from build123d import *

# Parameters (mm, degrees)
F0_R     = 11.425
F1_DEPTH = 8


with BuildPart() as f1:
    # F0 (on Front) → F1 (new body)
    with BuildSketch(Plane.XZ):
        with BuildLine():
            ThreePointArc((-40.4296863013, -48.1120131359), (-39.1212964763, -51.0311038498), (-38.6734638929, -54.1985034943))
            ThreePointArc((-38.6734638929, -54.1985034943), (-53.2658635374, -65.1756709109), (-59.7672414846, -48.1120131359))
            Line((-59.7672414846, -48.1120131359), (-65.0984638929, -49.8442323013))
            Line((-65.0984638929, -49.8442323013), (-65.0984638929, -54.1985034943))
            ThreePointArc((-65.0984638929, -54.1985034943), (-50.0984638929, -69.1985034943), (-35.0984638929, -54.1985034943))
            Line((-35.0984638929, -54.1985034943), (-35.0984638929, -49.8442323013))
            Line((-35.0984638929, -49.8442323013), (-40.4296863013, -48.1120131359))
        make_face()
        with BuildLine():
            ThreePointArc((-45.8538077773, -43.5912644821), (-42.7837389166, -45.4220905869), (-40.4296863013, -48.1120131359))
            Line((-40.4296863013, -48.1120131359), (-35.0984638929, -49.8442323013))
            Line((-35.0984638929, -49.8442323013), (-35.0984638929, -44.23865333))
            ThreePointArc((-35.0984638929, -44.23865333), (-36.9292899977, -41.1685844692), (-37.7218056429, -37.6830190937))
            Line((-37.7218056429, -37.6830190937), (-37.9632089773, -38.0152822786))
            ThreePointArc((-37.9632089773, -38.0152822786), (-41.2816851085, -41.3337584099), (-45.4632089773, -43.4643512387))
            Line((-45.4632089773, -43.4643512387), (-45.8538077773, -43.5912644821))
        make_face()
        with BuildLine():
            Line((-65.0984638929, -49.8442323013), (-59.7672414846, -48.1120131359))
            ThreePointArc((-59.7672414846, -48.1120131359), (-57.4131888693, -45.4220905869), (-54.3431200085, -43.5912644821))
            Line((-54.3431200085, -43.5912644821), (-54.7337188086, -43.4643512387))
            ThreePointArc((-54.7337188086, -43.4643512387), (-58.9152426773, -41.3337584099), (-62.2337188086, -38.0152822786))
            Line((-62.2337188086, -38.0152822786), (-62.4751221429, -37.6830190937))
            ThreePointArc((-62.4751221429, -37.6830190937), (-63.2676377882, -41.1685844692), (-65.0984638929, -44.23865333))
            Line((-65.0984638929, -44.23865333), (-65.0984638929, -49.8442323013))
        make_face()
        with BuildLine():
            Line((-35.0984638929, -44.23865333), (-35.0984638929, -49.8442323013))
            Line((-35.0984638929, -49.8442323013), (-30.9573059012, -51.1897760981))
            ThreePointArc((-30.9573059012, -51.1897760981), (-12.0562032411, -41.5591832693), (-21.6867960699, -22.6580806092))
            Line((-21.6867960699, -22.6580806092), (-25.8279540617, -21.3125368125))
            Line((-25.8279540617, -21.3125368125), (-29.1228307116, -25.8475454636))
            ThreePointArc((-29.1228307116, -25.8475454636), (-19.3030867945, -27.9092310939), (-14.8970509856, -36.9239283536))
            ThreePointArc((-14.8970509856, -36.9239283536), (-22.4323140065, -47.6663941429), (-35.0984638929, -44.23865333))
        make_face()
        with BuildLine():
            Line((-69.2396218847, -51.1897760981), (-65.0984638929, -49.8442323013))
            Line((-65.0984638929, -49.8442323013), (-65.0984638929, -44.23865333))
            ThreePointArc((-65.0984638929, -44.23865333), (-84.740697499, -40.4544475144), (-71.0740970743, -25.8475454636))
            Line((-71.0740970743, -25.8475454636), (-74.3689737242, -21.3125368125))
            Line((-74.3689737242, -21.3125368125), (-78.5101317159, -22.6580806092))
            ThreePointArc((-78.5101317159, -22.6580806092), (-88.1407245447, -41.5591832693), (-69.2396218847, -51.1897760981))
        make_face()
        with BuildLine():
            Line((-74.3689737242, -21.3125368125), (-71.0740970743, -25.8475454636))
            ThreePointArc((-71.0740970743, -25.8475454636), (-67.7883864419, -27.255150762), (-65.0984638929, -29.6092033773))
            Line((-65.0984638929, -29.6092033773), (-65.0984638929, -29.1985034943))
            ThreePointArc((-65.0984638929, -29.1985034943), (-64.3643116374, -24.5632485786), (-62.2337188086, -20.3817247099))
            Line((-62.2337188086, -20.3817247099), (-61.9923154742, -20.0494615249))
            ThreePointArc((-61.9923154742, -20.0494615249), (-65.5521859403, -20.3728332923), (-69.0377513159, -19.580317647))
            Line((-69.0377513159, -19.580317647), (-74.3689737242, -21.3125368125))
        make_face()
        with BuildLine():
            Line((-35.0984638929, -29.1985034943), (-35.0984638929, -29.6092033773))
            ThreePointArc((-35.0984638929, -29.6092033773), (-32.408541344, -27.255150762), (-29.1228307116, -25.8475454636))
            Line((-29.1228307116, -25.8475454636), (-25.8279540617, -21.3125368125))
            Line((-25.8279540617, -21.3125368125), (-31.15917647, -19.580317647))
            ThreePointArc((-31.15917647, -19.580317647), (-34.6447418456, -20.3728332923), (-38.2046123117, -20.0494615249))
            Line((-38.2046123117, -20.0494615249), (-37.9632089773, -20.3817247099))
            ThreePointArc((-37.9632089773, -20.3817247099), (-35.8326161485, -24.5632485786), (-35.0984638929, -29.1985034943))
        make_face()
        with BuildLine():
            Line((-31.15917647, -19.580317647), (-25.8279540617, -21.3125368125))
            Line((-25.8279540617, -21.3125368125), (-23.26857767, -17.7898574193))
            ThreePointArc((-23.26857767, -17.7898574193), (-26.5870538012, 3.1621762807), (-47.5390875012, -0.1562998505))
            Line((-47.5390875012, -0.1562998505), (-50.0984638929, -3.6789792437))
            Line((-50.0984638929, -3.6789792437), (-46.803587243, -8.2139878949))
            ThreePointArc((-46.803587243, -8.2139878949), (-35.0240773753, 2.4456082853), (-23.9788325856, -8.9730786349))
            ThreePointArc((-23.9788325856, -8.9730786349), (-25.9427063017, -15.3775859883), (-31.15917647, -19.580317647))
        make_face()
        with BuildLine():
            Line((-76.9283501159, -17.7898574193), (-74.3689737242, -21.3125368125))
            Line((-74.3689737242, -21.3125368125), (-69.0377513159, -19.580317647))
            ThreePointArc((-69.0377513159, -19.580317647), (-71.5085417077, 0.2699405258), (-53.3933405429, -8.2139878949))
            Line((-53.3933405429, -8.2139878949), (-50.0984638929, -3.6789792437))
            Line((-50.0984638929, -3.6789792437), (-52.6578402846, -0.1562998505))
            ThreePointArc((-52.6578402846, -0.1562998505), (-73.6098739846, 3.1621762807), (-76.9283501159, -17.7898574193))
        make_face()
        with BuildLine():
            Line((-50.0984638929, -3.6789792437), (-53.3933405429, -8.2139878949))
            ThreePointArc((-53.3933405429, -8.2139878949), (-53.3744082801, -8.5933234246), (-53.3680952002, -8.9730786349))
            ThreePointArc((-53.3680952002, -8.9730786349), (-53.8159277836, -12.1404782793), (-55.1243176086, -15.0595689933))
            Line((-55.1243176086, -15.0595689933), (-54.7337188086, -14.9326557498))
            ThreePointArc((-54.7337188086, -14.9326557498), (-50.0984638929, -14.1985034943), (-45.4632089773, -14.9326557498))
            Line((-45.4632089773, -14.9326557498), (-45.0726101773, -15.0595689933))
            ThreePointArc((-45.0726101773, -15.0595689933), (-46.4802154756, -11.773858361), (-46.803587243, -8.2139878949))
            Line((-46.803587243, -8.2139878949), (-50.0984638929, -3.6789792437))
        make_face()
        with BuildLine():
            ThreePointArc((-54.3346800554, -43.5878909943), (-50.0984638929, -42.7735034943), (-45.8622477305, -43.5878909943))
            ThreePointArc((-45.8622477305, -43.5878909943), (-45.6622982862, -43.5275102536), (-45.4632089773, -43.4643512387))
            ThreePointArc((-45.4632089773, -43.4643512387), (-41.2816851085, -41.3337584099), (-37.9632089773, -38.0152822786))
            ThreePointArc((-37.9632089773, -38.0152822786), (-37.8416192047, -37.845454303), (-37.7224059316, -37.6739497561))
            ThreePointArc((-37.7224059316, -37.6739497561), (-37.1878716842, -33.3934091929), (-35.1042803595, -29.6161877847))
            ThreePointArc((-35.1042803595, -29.6161877847), (-35.0999180801, -29.4073658878), (-35.0984638929, -29.1985034943))
            ThreePointArc((-35.0984638929, -29.1985034943), (-35.8326161485, -24.5632485786), (-37.9632089773, -20.3817247099))
            ThreePointArc((-37.9632089773, -20.3817247099), (-38.0871516741, -20.2136062338), (-38.2134232637, -20.0472298539))
            ThreePointArc((-38.2134232637, -20.0472298539), (-42.1192790931, -18.2160977956), (-45.0677649982, -15.0672590823))
            ThreePointArc((-45.0677649982, -15.0672590823), (-45.2650184055, -14.9985807931), (-45.4632089773, -14.9326557498))
            ThreePointArc((-45.4632089773, -14.9326557498), (-50.0984638929, -14.1985034943), (-54.7337188086, -14.9326557498))
            ThreePointArc((-54.7337188086, -14.9326557498), (-54.9319093804, -14.9985807931), (-55.1291627877, -15.0672590823))
            ThreePointArc((-55.1291627877, -15.0672590823), (-58.0776486928, -18.2160977956), (-61.9835045222, -20.0472298539))
            ThreePointArc((-61.9835045222, -20.0472298539), (-62.1097761118, -20.2136062338), (-62.2337188086, -20.3817247099))
            ThreePointArc((-62.2337188086, -20.3817247099), (-64.3643116374, -24.5632485786), (-65.0984638929, -29.1985034943))
            ThreePointArc((-65.0984638929, -29.1985034943), (-65.0970097058, -29.4073658878), (-65.0926474263, -29.6161877847))
            ThreePointArc((-65.0926474263, -29.6161877847), (-63.1308646168, -33.0384647775), (-62.4498768003, -36.9239283536))
            ThreePointArc((-62.4498768003, -36.9239283536), (-62.456039726, -37.299141454), (-62.4745218543, -37.6739497561))
            ThreePointArc((-62.4745218543, -37.6739497561), (-62.3553085811, -37.845454303), (-62.2337188086, -38.0152822786))
            ThreePointArc((-62.2337188086, -38.0152822786), (-58.9152426773, -41.3337584099), (-54.7337188086, -43.4643512387))
            ThreePointArc((-54.7337188086, -43.4643512387), (-54.5346294996, -43.5275102536), (-54.3346800554, -43.5878909943))
        make_face()
        with Locations((-50.0984638929, -29.1985034943)):
            Circle(F0_R, mode=Mode.SUBTRACT)
    extrude(amount=F1_DEPTH)


solid = f1.part
Source: CAD feature listing. Evaluate the final solid. Frame: model axes, mm. A direction names the side the tool comes from. Give positions to 0.01 mm unless a question says otherwise; leave off trailing zeros. Write each loop counter-clockwise with the first axis right and the second up, starting at its lowest first coordinate (ties: lowest second). Pieces come first, ordered by that corner, then holes. Notation, with made-up numbers: M 68,-6 L 106,-6 A21 ccw 106,18 Z; hole C 30,0.25 d10. An arc over 180 degrees is marked long. Return JSON: item names as keys, results as strings. Group by question number.
1) Cut plane C-C, the plane z = -10.5. Output: boundary loops of the cut face in (x, y).
2) Pin query (flat end, axial travel): P1, Ø3, axis at y = -3.5, z = -23, coming from the -X side; P2, Ø1, axis at y = -6, z = -7.5, coming from the -X side; P3, Ø3.5, axis at y = -4.5, z = -52, coming from the +X side. Return the tip coordinate at first contact, or that it passes through.
3) Pull-direction query (Z, two-part tool) for faces 1 (the face through (-50.159, -3.944, -42.774)), 2 (the face through (-67.198, -3.944, -50.526)), 3 (the face through (-48.8, -3.94, -1.89)); classes: pulls with the +Z half, pulls with the -Z half, needs draft (parallel to the pull), parting line crosses it, or undercut.
4) Cut plane B-B, the plane x = -49. Output: boundary loops of the cut face in (y, z), plus the area to 3 significant figures.
5) Cut plane D-D, the plane y = -2.5. Give the number of separate pieces and of enclosed holes in the cut face, plus the area to 3 significant figures.
6) Set-up query: faces 4 (the face through (-51.36, -3.94, -1.94)), 5 (the face through (-37.206, -3.944, -33.451)), 6 (the face through (-75.667, -3.944, -19.527)), 7 (the face through (-35.098, -4, -52)). Return all of +Z, -Z, +X, -X, +Y, -Y with unobstructed straight access to the full face (end or side cutting, diameter ignored); none if empty.
7) Material intervals for line 1 along X through (y, z) = (-2.25, -53.5); line 2 along X through (y, z) = (-0.5, -34.5); line 3 along Z through (x, y) = (-69, -7), sorted ascending. Write a range as [from, to].
8) Cut plane A-A, the plane z = -32. Output: boundary loops of the cut face in (x, y), plus the area to 3 significant figures.
Recorded:
{
 "1": {"outline": "M -79.72,-8 L -76.12,-8 L -76.12,0 L -79.72,0 Z; M -53.47,-8 L -46.73,-8 L -46.73,0 L -53.47,0 Z; M -24.08,-8 L -20.48,-8 L -20.48,0 L -24.08,0 Z"},
 "2": {"P1": "stops at x = -82.28", "P2": "stops at x = -79.76", "P3": "stops at x = -19.44"},
 "3": {"face 1": "undercut", "face 2": "pulls with the -Z half", "face 3": "pulls with the +Z half"},
 "4": {"outline": "M -8,-69.16 L 0,-69.16 L 0,-65.57 L -8,-65.57 Z; M -8,-42.83 L 0,-42.83 L 0,-40.57 L -8,-40.57 Z; M -8,-17.83 L 0,-17.83 L 0,-2.17 L -8,-2.17 Z", "area": "172 mm²"},
 "5": {"separate pieces": "1", "enclosed holes": "6", "area": "1,510 mm²"},
 "6": {"face 4": "+Z, +Y, -Y", "face 5": "+Y, -Y", "face 6": "-X, +Y, -Y", "face 7": "-Z, +Y, -Y"},
 "7": {"line 1": "x = [-65.1, -61.5], [-38.69, -35.1]", "line 2": "x = [-88.68, -85.04], [-62.71, -60.22], [-39.98, -37.49], [-15.16, -11.52]", "line 3": "z = [-51.11, -47.26], [-26.59, -19.6], [1.65, 5.42]"},
 "8": {"outline": "M -88.04,-8 L -84.18,-8 L -84.18,0 L -88.04,0 Z; M -63.57,-8 L -61.17,-8 L -61.17,0 L -63.57,0 Z; M -39.02,-8 L -36.63,-8 L -36.63,0 L -39.02,0 Z; M -16.01,-8 L -12.15,-8 L -12.15,0 L -16.01,0 Z", "area": "100 mm²"}
}
